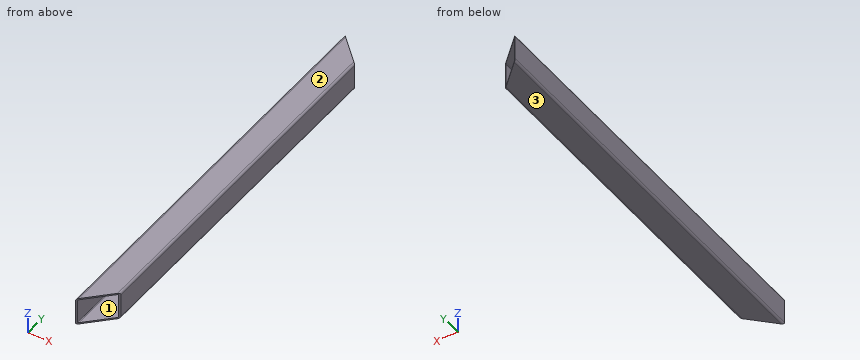
from build123d import *

# Parameters (mm, degrees)
F2_W     = 40
F2_H     = 40
F3_DEPTH = 300
F4_R     = 3
F5_T     = -2
F7_DEPTH = 40.001


with BuildPart() as f3:
    # F2 (on Front) → F3 (new body, symmetric)
    with BuildSketch(Plane.XZ):
        Rectangle(F2_W, F2_H)
    extrude(amount=F3_DEPTH, both=True)

    # F4
    f4_edges = [f3.edges().sort_by_distance(p)[0] for p in [
        (20, 0, 20),
        (-20, 0, 20),
        (20, 0, -20),
        (-20, 0, -20),
    ]]
    fillet(f4_edges, radius=F4_R)

    # F5
    f5_openings = [f3.faces().sort_by_distance(p)[0] for p in [
        (0, -300, 0),
        (0, 300, 0),
    ]]
    offset(amount=F5_T, openings=f5_openings)

    # F6 (on face) → F7 (cut, through all)
    with BuildSketch(Plane.XY.offset(20)):
        Polygon((20, -300), (20, -260), (-20, -300), align=None)
        Polygon((20, 300), (-20, 300), (20, 260), align=None)
    extrude(amount=-F7_DEPTH, mode=Mode.SUBTRACT)


solid = f3.part
Geometry: final body of the model. Coordinates: model frame, mm. Face numbers are marked on the shaded views. Round coordinates to 2 decimals unless told otherwise and drop trailing zeros. Loops run counter-clockwise (first coordinate to the right, second up) from the corner with the lowest first, then second, coordinate; pieces in that order, holes last. Notation, with made-up numbers: (59.25, 11.25) -> (100.25, 11.25) arc R26 ccw to (100.25, 34.25) -> close; hole circle Ø6 at (48, 1.25). An arc over 180 degrees is marked (long way). One line per question, with ' | ' between items. Start each with the question number.
1. Line query: line 1 along X through (y, z) = (251, 8). Output: solid intervals per line, ascending. Write a range as [from, to].
2. Section C-C on z = 9. Output: boundary loops of the cut face in (x, y).
3. Mould query, pull axis Z, two halves, no side actions, for the marked faces 1, 2 and 3. Classes: pulls with the +Z half, pulls with the -Z half, needs draft (parallel to the pull), parting line crosses it, or undercut.
4. Section B-B on y = 62. Output: boundary loops of the cut face in (x, z), and give its area (3 significant figures).
5. Section A-A on x = 3. Output: boundary loops of the cut face in (y, z), and give its area (3 significant figures).
Returned:
1) line 1: x = [-20, -18], [18, 20]
2) outline: (-20, -300) -> (-18, -298) -> (-18, 298) -> (-20, 300) -> close; (18, -262) -> (20, -260) -> (20, 260) -> (18, 262) -> close
3) face 1: undercut | face 2: pulls with the +Z half | face 3: pulls with the -Z half
4) outline: (-20, -17) arc R3 ccw to (-17, -20) -> (17, -20) arc R3 ccw to (20, -17) -> (20, 17) arc R3 ccw to (17, 20) -> (-17, 20) arc R3 ccw to (-20, 17) -> close; hole (-18, -17) arc R1 ccw to (-17, -18) -> (17, -18) arc R1 ccw to (18, -17) -> (18, 17) arc R1 ccw to (17, 18) -> (-17, 18) arc R1 ccw to (-18, 17) -> close | area: 297 mm2
5) outline: (-277, -20) -> (277, -20) -> (277, -18) -> (-277, -18) -> close; (-277, 18) -> (277, 18) -> (277, 20) -> (-277, 20) -> close | area: 2,220 mm2
